```python
from build123d import *

# Parameters (mm, degrees)
ESQUISSE1_W             = 25
ESQUISSE1_H             = 75
BOSS_EXTRU_1_DEPTH      = 51
ESQUISSE2_R             = 3.5
ENL_V_MAT_EXTRU_1_DEPTH = 70
ESQUISSE3_W             = 15
ESQUISSE3_H             = 41
ENL_V_MAT_EXTRU_2_DEPTH = 29
ESQUISSE4_R             = 1.75
ESQUISSE4_R_2           = 1.5
ENL_V_MAT_EXTRU_3_DEPTH = 25


with BuildPart() as part:
    # Esquisse1 → Boss.-Extru.1 (new body)
    with BuildSketch(Plane.XY):
        with Locations((5.975, -32.109782609)):
            Rectangle(ESQUISSE1_W, ESQUISSE1_H)
    extrude(amount=BOSS_EXTRU_1_DEPTH)

    # Esquisse2 → Enlèv. mat.-Extru.1 (cut)
    with BuildSketch(Plane.XY.offset(51)):
        with Locations((5.975, -51.609782609)):
            Circle(ESQUISSE2_R)
    extrude(amount=-ENL_V_MAT_EXTRU_1_DEPTH, mode=Mode.SUBTRACT)

    # Esquisse3 → Enlèv. mat.-Extru.2 (cut)
    with BuildSketch(Plane.XZ.offset(69.609782609)):
        with Locations((5.975, 25.5)):
            Rectangle(ESQUISSE3_W, ESQUISSE3_H)
    extrude(amount=-ENL_V_MAT_EXTRU_2_DEPTH, mode=Mode.SUBTRACT)

    # Esquisse4 → Enlèv. mat.-Extru.3 (cut)
    with BuildSketch(Plane(origin=(18.475, 0, 0), x_dir=(0, 0, -1), z_dir=(1, 0, 0))):
        with Locations(Location((-46, -4.609782609, 0), (0, 0, 90))):
            Circle(ESQUISSE4_R)
        with Locations(Location((-5, -4.609782609, 0), (0, 0, 90))):
            Circle(ESQUISSE4_R_2)
    extrude(amount=-ENL_V_MAT_EXTRU_3_DEPTH, mode=Mode.SUBTRACT)


solid = part.part
```
Verification items for the finished model (mm, model axes). A direction names the side the tool comes from. Give positions to 0.01 mm unless a question says otherwise; leave off trailing zeros. Order: outer loops, then holes, each group sorted by start corner. A loop starts at its lowest first (then second) coordinate and runs counter-clockwise, first axis right, second up. Notation, with made-up numbers: (40, -19) -> (75, -19) arc R26 cw to (75, 7) -> close; hole circle Ø3 at (15.25, -19.5). An arc over 180 degrees is marked (long way). One line per item, written item: value.
(1) Sectioned sample at C-C on y = -46.5. Record the cut outline in (x, z) (3 decimals), then the cut area to 3 significant figures.
Final values:
outline: (-6.525, 0) -> (18.475, 0) -> (18.475, 51) -> (-6.525, 51) -> close; hole (-1.525, 5) -> (13.475, 5) -> (13.475, 46) -> (-1.525, 46) -> close
area: 660 mm^2
(2) Sectioned sample at D-D on z = 29. Record the cut outline in (x, y) (3 decimals).
Final values:
outline: (-6.525, -69.61) -> (-1.525, -69.61) -> (-1.525, -40.61) -> (13.475, -40.61) -> (13.475, -69.61) -> (18.475, -69.61) -> (18.475, 5.39) -> (-6.525, 5.39) -> close
(3) Draft check along Y on faces 1 (the face through (-6.525, -33, 25)), 2 (the face through (6.15, -4.99, 44.29)), 3 (the face through (7.59, -54.715, 2.535)), 4 (the face through (6, 5.39, 25)). Enter one of: pulls with the +Y half, pulls with the -Y half, needs draft (parallel to the pull), parting line crosses it, or undercut.
Final values:
face 1: needs draft
face 2: undercut
face 3: undercut
face 4: pulls with the +Y half
(4) Tool access check on faces 5 (the face through (-1.525, -55, 25)), 6 (the face through (-3, -69.61, 25)). Record the directions out of +Z, -Z, +X, -X, +Y, -Y that give a thin tool (end or side, any length) a straight path to the whole face; none if there is none.
Final values:
face 5: -Y
face 6: +Z, -Z, +X, -X, -Y
(5) Sectioned sample at A-A on x = 12. Record the cut outline in (y, z).
Final values:
outline: (-69.61, 0) -> (5.39, 0) -> (5.39, 51) -> (-69.61, 51) -> (-69.61, 46) -> (-40.61, 46) -> (-40.61, 5) -> (-69.61, 5) -> close; hole circle Ø3.5 at (-4.61, 46); hole circle Ø3 at (-4.61, 5)
(6) Scan lines: line 1 along Z through (x, y) = (12, -58); line 2 along X through (y, z) = (-49.5, 34.5) (3 decimals); line 3 along Y through (x, z) = (4.5, 36). Record each from-to range of solid material in increasing order. Write a range as [from, to].
Final values:
line 1: [0, 5], [46, 51]
line 2: [-6.525, -1.525], [13.475, 18.475]
line 3: [-40.61, 5.39]
(7) Gauge pin test, flat end, axial feed: pin 1 (12 mm diameter, centred on x = 5, z = 17.5, fed in from -Y). Record the tip position at first contact, or that the pin passes through.
Final values:
pin 1: y = -40.61
(8) Sectioned sample at B-B on x = 5.75. Record the cut outline in (y, z), then the cut area to 3 significant figures.
Final values:
outline: (-69.61, 0) -> (-55.1, 0) -> (-55.1, 5) -> (-69.61, 5) -> close; (-69.61, 46) -> (-55.1, 46) -> (-55.1, 51) -> (-69.61, 51) -> close; (-48.12, 0) -> (5.39, 0) -> (5.39, 51) -> (-48.12, 51) -> (-48.12, 46) -> (-40.61, 46) -> (-40.61, 5) -> (-48.12, 5) -> close; hole circle Ø3.5 at (-4.61, 46); hole circle Ø3 at (-4.61, 5)
area: 2,550 mm^2
